Study the drawing (mm; zero at the part's minimum x, y, z) and answer. A direction names the side the tool comes from. Round coordinates to 2 decimals unless told otherwise and drop trailing zeros. Order: outer loops, then holes, each group sorted by start corner. A loop starts at its lowest first (then second) coordinate and runs counter-clockwise, first axis right, second up. Notation, with made-up numbers: (-28.75, 14) - (-13.75, 14) arc R9 cw to (-13.75, 25) - close; hole circle Ø9 at (58.5, 84.5). An arc over 180 degrees is marked (long way). Put each result on its own line as item: value.
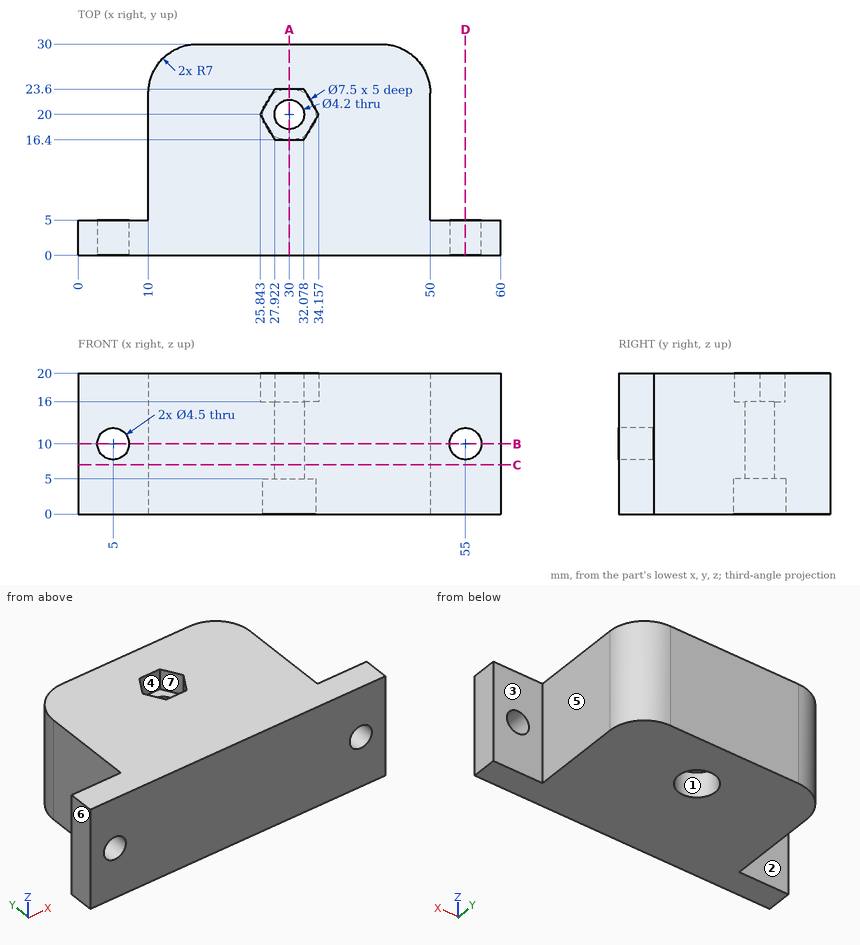
1) For a pull along X with two mould halves and no side action, classify the marked faces 4, 5, 6 and 7 as pulls with the +X half, pulls with the -X half, needs draft (parallel to the pull), parting line crosses it, or undercut.
Findings below:
face 4: undercut
face 5: pulls with the +X half
face 6: pulls with the -X half
face 7: undercut
2) A cutting plane is placed at D-D on x = 55. Write down the section's boundary in (y, z), then the cut area to 3 significant figures.
Findings below:
outline: (0, 0) - (5, 0) - (5, 7.75) - (0, 7.75) - close; (0, 12.25) - (5, 12.25) - (5, 20) - (0, 20) - close
area: 77.5 mm2
3) For the marked faces 1, 2 and 3, determine the directions among +Z, -Z, +X, -X, +Y, -Y from which every point of the face is accessible in a straight line to the end or side of a thin tool.
Findings below:
face 1: -Z
face 2: +Z, -Z, -X, +Y
face 3: +Z, -Z, +X, +Y
4) A cutting plane is placed at A-A on x = 30. Write down the section's boundary in (y, z).
Findings below:
outline: (0, 0) - (16.25, 0) - (16.25, 5) - (17.9, 5) - (17.9, 16) - (16.4, 16) - (16.4, 20) - (0, 20) - close; (22.1, 5) - (23.75, 5) - (23.75, 0) - (30, 0) - (30, 20) - (23.6, 20) - (23.6, 16) - (22.1, 16) - close
5) A cutting plane is placed at B-B on z = 10. Write down the section's boundary in (x, y), then the cut area to 3 significant figures.
Findings below:
outline: (0, 0) - (2.75, 0) - (2.75, 5) - (0, 5) - close; (7.25, 0) - (52.75, 0) - (52.75, 5) - (50, 5) - (50, 23) arc R7 ccw to (43, 30) - (17, 30) arc R7 ccw to (10, 23) - (10, 5) - (7.25, 5) - close; (57.25, 0) - (60, 0) - (60, 5) - (57.25, 5) - close; hole circle Ø4.2 at (30, 20)
area: 1,220 mm2
6) Given pin 1 Ø2 at (x, y) = (29.5, 21.5) entering from -Z; pin 2 Ø9 at (y, z) = (16, 9) entering from -X; pin 3 Ø4 at (x, z) = (5, 10) entering from -Y; pin 4 Ø12 at (y, z) = (17, 14.5) entering from +X, each flat-ended and moving along its own axis, determine where each tip first touches the part or whether it passes through.
Findings below:
pin 1: stops at z = 5
pin 2: stops at x = 10
pin 3: passes through
pin 4: stops at x = 50
7) A cutting plane is placed at C-C on z = 7. Write down the section's boundary in (x, y).
Findings below:
outline: (0, 0) - (60, 0) - (60, 5) - (50, 5) - (50, 23) arc R7 ccw to (43, 30) - (17, 30) arc R7 ccw to (10, 23) - (10, 5) - (0, 5) - close; hole circle Ø4.2 at (30, 20)
8) Straight lines are drawn through the part: L1, parallel to X at y = 3.65, z = 10; L2, parallel to Z at x = 5, y = 3.4; L3, parallel to X at y = 23, z = 14. For each, find the intervals that lie inside material, in ascending order. Write a range as from..to.
Findings below:
L1: x = 0..2.75, 7.25..52.75, 57.25..60
L2: z = 0..7.75, 12.25..20
L3: x = 10..50
